```python
from build123d import *

# Parameters (mm, degrees)
BOSS_EXTRUDE3_DEPTH = 1.6
SKETCH1_9_R         = 1.25
CUT_EXTRUDE2_DEPTH  = 1.6


with BuildPart() as part:
    # Sketch1 → Boss-Extrude3 (new body)
    with BuildSketch(Plane(origin=(0, 0, 0), x_dir=(1, 0, 0), z_dir=(0, 1, 0))):
        with BuildLine():
            Line((-30, -39), (-30, -6))
            Line((-30, -6), (-25, -6))
            ThreePointArc((-25, -6), (-19, 0), (-25, 6))
            Line((-25, 6), (-30, 6))
            Line((-30, 6), (-30, 39))
            Line((-30, 39), (-24, 39))
            ThreePointArc((-24, 39), (-19.757359313, 40.757359313), (-18, 45))
            Line((-18, 45), (-18, 54))
            Line((-18, 54), (18, 54))
            Line((18, 54), (18, 45))
            ThreePointArc((18, 45), (19.757359313, 40.757359313), (24, 39))
            Line((24, 39), (30, 39))
            Line((30, 39), (30, 6))
            Line((30, 6), (25, 6))
            ThreePointArc((25, 6), (19, 0), (25, -6))
            Line((25, -6), (30, -6))
            Line((30, -6), (30, -39))
            Line((30, -39), (24, -39))
            ThreePointArc((24, -39), (19.757359313, -40.757359313), (18, -45))
            Line((18, -45), (18, -54))
            Line((18, -54), (-18, -54))
            Line((-18, -54), (-18, -45))
            ThreePointArc((-18, -45), (-19.757359313, -40.757359313), (-24, -39))
            Line((-24, -39), (-30, -39))
        make_face()
    extrude(amount=BOSS_EXTRUDE3_DEPTH)

    # Sketch1_9 → Cut-Extrude2 (cut)
    with BuildSketch(Plane(origin=(0, 0, 0), x_dir=(1, 0, 0), z_dir=(0, 1, 0))):
        with Locations(Location((-27.5, -35, 0), (0, 0, 270))):
            Circle(SKETCH1_9_R)
        with Locations(Location((-27.5, -10, 0), (0, 0, 270))):
            Circle(SKETCH1_9_R)
        with Locations(Location((27.5, -10, 0), (0, 0, 270))):
            Circle(SKETCH1_9_R)
        with Locations(Location((27.5, -35, 0), (0, 0, 270))):
            Circle(SKETCH1_9_R)
        with Locations(Location((27.5, 35, 0), (0, 0, 270))):
            Circle(SKETCH1_9_R)
        with Locations(Location((-27.5, 35, 0), (0, 0, 270))):
            Circle(SKETCH1_9_R)
    extrude(amount=CUT_EXTRUDE2_DEPTH, mode=Mode.SUBTRACT)


solid = part.part
```
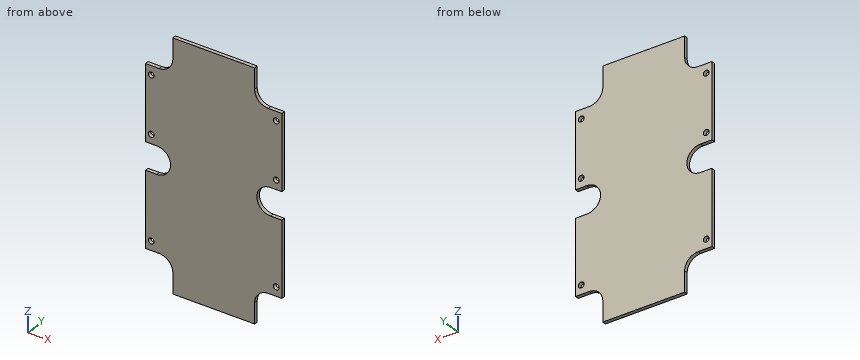
Source: CAD feature listing. Evaluate the final solid. Frame: model axes, mm. Coordinates: 2 decimals unless noted, no trailing zeros. Order: outer loops, then holes, each group sorted by start corner. A loop starts at its lowest first (then second) coordinate and runs counter-clockwise, first axis right, second up. Notation, with made-up numbers: M 17.5,22 L 59.5,22 A18 ccw 59.5,45 Z; hole C -8,85 d9. An arc over 180 degrees is marked long. Write each question's results on one line, items separated by ' | '. Start each with the question number.
1) Section query B-B (x = -27.5). Return the cut outline in (y, z).
2) Line query: line 1 (X direction, y = 1.2, z = 10); line 2 (Z direction, x = -24.5, y = 0.1); line 3 (X direction, y = 0.9, z = -34.5). Output: solid intervals per line, ascending. Write a range as from..to.
3) Section query D-D (x = 21). Return the cut outline in (y, z), plus the area to 3 significant figures.
4) Contact query for flat-ended pins moving along their axis: pin 1 Ø2 at (x, z) = (27.5, 35) entering from -Y; pin 2 Ø0.8 at (x, y) = (-27, 1) entering from +Z; pin 3 Ø0.8 at (y, z) = (1, 49.5) entering from +X; pin 4 Ø0.5 at (x, y) = (-27.5, 1) entering from -Z. Output: stop coordinate, or through.
5) Section query A-A (y = 0.25). Give the number of separate pieces and of enclosed holes in the cut face, plus the area to 3 significant figures.
6) Section query C-C (z = 10). Return the cut outline in (x, y), plus the area to 3 significant figures.
Answers:
1) outline: M 0,-39 L 1.6,-39 L 1.6,-36.25 L 0,-36.25 Z; M 0,-33.75 L 1.6,-33.75 L 1.6,-6 L 0,-6 Z; M 0,6 L 1.6,6 L 1.6,8.75 L 0,8.75 Z; M 0,11.25 L 1.6,11.25 L 1.6,33.75 L 0,33.75 Z; M 0,36.25 L 1.6,36.25 L 1.6,39 L 0,39 Z
2) line 1: x = -30..-28.75, -26.25..26.25, 28.75..30 | line 2: z = -39..-5.98, 5.98..39 | line 3: x = -30..-28.65, -26.35..26.35, 28.65..30
3) outline: M 0,-39.8 L 1.6,-39.8 L 1.6,-4.47 L 0,-4.47 Z; M 0,4.47 L 1.6,4.47 L 1.6,39.8 L 0,39.8 Z | area: 113 mm^2
4) pin 1: passes through | pin 2: stops at z = 39 | pin 3: stops at x = 18 | pin 4: stops at z = -39
5) separate pieces: 1 | enclosed holes: 6 | area: 5,530 mm^2
6) outline: M -30,0 L -28.75,0 L -28.75,1.6 L -30,1.6 Z; M -26.25,0 L 26.25,0 L 26.25,1.6 L -26.25,1.6 Z; M 28.75,0 L 30,0 L 30,1.6 L 28.75,1.6 Z | area: 88.0 mm^2
